from build123d import *

# Parameters (mm, degrees)
SKETCH1_W           = 38.1
SKETCH1_H           = 304.8
BOSS_EXTRUDE1_DEPTH = 6.35
SKETCH2_W           = 6.35
SKETCH2_H           = 25.4
CUT_EXTRUDE1_DEPTH  = 7.35


with BuildPart() as part:
    # Sketch1 → Boss-Extrude1 (new body)
    with BuildSketch(Plane.XY):
        Rectangle(SKETCH1_W, SKETCH1_H)
    extrude(amount=BOSS_EXTRUDE1_DEPTH)

    # Sketch2 → Cut-Extrude1 (cut, through all)
    with BuildSketch(Plane.XY.offset(6.35)):
        with Locations((0, 127)):
            Rectangle(SKETCH2_W, SKETCH2_H)
    cut_extrude1 = extrude(amount=-CUT_EXTRUDE1_DEPTH, mode=Mode.SUBTRACT)

    # Mirror1: Cut-Extrude1 across plane
    add(cut_extrude1.mirror(Plane.ZX), mode=Mode.SUBTRACT)


solid = part.part
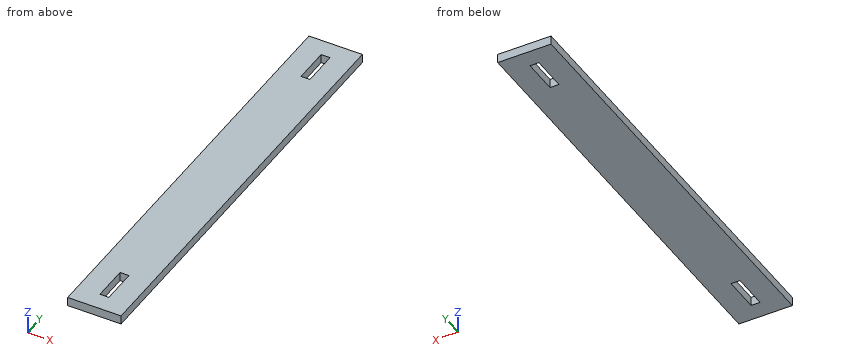
Geometry check sheet. Reference: the model listing, model coordinates, mm. Give positions to 0.01 mm unless a question says otherwise; leave off trailing zeros. Loops run counter-clockwise (first coordinate to the right, second up) from the corner with the lowest first, then second, coordinate; pieces in that order, holes last.
(1) Section check A-A on x = -0.5. Record the cut outline in (y, z), then the cut area to 3 significant figures.
From the geometry:
outline: (-152.4, 0) - (-139.7, 0) - (-139.7, 6.35) - (-152.4, 6.35) - close; (-114.3, 0) - (114.3, 0) - (114.3, 6.35) - (-114.3, 6.35) - close; (139.7, 0) - (152.4, 0) - (152.4, 6.35) - (139.7, 6.35) - close
area: 1,610 mm2
(2) Section check C-C on y = -124.5. Record the cut outline in (x, z) (3 decimals).
From the geometry:
outline: (-19.05, 0) - (-3.175, 0) - (-3.175, 6.35) - (-19.05, 6.35) - close; (3.175, 0) - (19.05, 0) - (19.05, 6.35) - (3.175, 6.35) - close
(3) Thickness scan on L1, parallel to Y at x = -1.5, z = 1. Record the ranges inside material, lowest first.
From the geometry:
L1: y = -152.4 to -139.7, -114.3 to 114.3, 139.7 to 152.4
(4) Section check B-B on z = 1.75. Record the cut outline in (x, y) (3 decimals), then the cut area to 3 significant figures.
From the geometry:
outline: (-19.05, -152.4) - (19.05, -152.4) - (19.05, 152.4) - (-19.05, 152.4) - close; hole (-3.175, -139.7) - (3.175, -139.7) - (3.175, -114.3) - (-3.175, -114.3) - close; hole (-3.175, 114.3) - (3.175, 114.3) - (3.175, 139.7) - (-3.175, 139.7) - close
area: 11,300 mm2
